from build123d import *

# Parameters (mm, degrees)
F0_W     = 181
F0_H     = 181
F0_W_2   = 20
F0_H_2   = 120
F1_DEPTH = 3


with BuildPart() as f1:
    # F0 (on Right) → F1 (new body)
    with BuildSketch(Plane.YZ):
        Rectangle(F0_W, F0_H)
        Polygon((8.017361, -22.155164), (10.511788, -22.155164), (11.657102, -24.445793), (13.264574, -44.539195), (13.264574, -24.155164), (19.664574, -24.155164), (19.664574, -27.155164), (24.664574, -27.155164), (24.664574, -72.955163), (3.864575, -72.955163), (3.864575, -27.155164), (8.864575, -27.155164), (8.864575, -24.955163), (6.617362, -24.955163), align=None, mode=Mode.SUBTRACT)
        Polygon((31.895746, -73.251659), (31.895746, -27.251661), (36.895746, -27.251661), (36.895746, -25.251659), (34.586729, -25.251659), (36.086728, -22.251661), (38.70476, -22.251661), (39.886403, -24.614947), (41.395744, -43.481709), (41.395744, -24.251661), (47.895743, -24.251661), (47.895743, -27.251661), (52.895743, -27.251661), (52.895743, -73.251659), align=None, mode=Mode.SUBTRACT)
        Polygon((73.728273, -23.606915), (73.728273, -26.606915), (78.728273, -26.606915), (78.728273, -72.806911), (57.528277, -72.806911), (57.528277, -26.606915), (62.528277, -26.606915), (62.528277, -24.806911), (60.157458, -24.806911), (61.757456, -21.606915), (64.499095, -21.606915), (65.717066, -24.042858), (67.128275, -41.682975), (67.128275, -23.606915), align=None, mode=Mode.SUBTRACT)
        with Locations((-69.899997, 23.899991)):
            Rectangle(F0_W_2, F0_H_2, mode=Mode.SUBTRACT)
        Polygon((-51.186814, -46.700009), (-51.186814, 83.899991), (-33.861232, 83.899991), (-33.861232, 73.899991), (-40.861232, 73.899991), (-40.861232, 63.999991), (-33.400224, 63.999991), (-33.400224, 53.799991), (-40.861232, 53.799991), (-40.861232, 44.099991), (-33.300224, 44.099991), (-33.300224, 33.699991), (-40.861232, 33.699991), (-40.861232, 24.199991), (-33.200224, 24.199991), (-33.200224, 13.599991), (-40.861232, 13.599991), (-40.861232, 4.299991), (-32.686683, 4.299991), (-32.686683, -6.500009), (-40.861232, -6.500009), (-40.861232, -15.600009), (-31.84899, -15.600009), (-31.84899, -26.600009), (-40.861232, -26.600009), (-40.861232, -35.500009), (-31.998828, -35.500009), (-31.998828, -46.700009), align=None, mode=Mode.SUBTRACT)
        Polygon((-7.774414, 73.899968), (-14.774414, 73.899968), (-14.774414, 63.799968), (-7.513406, 63.799968), (-7.513406, 53.999968), (-14.774414, 53.999968), (-14.774414, 43.699968), (-7.613406, 43.699968), (-7.613406, 34.099968), (-14.774414, 34.099968), (-14.774414, 23.599968), (-7.713406, 23.599968), (-7.713406, 14.199968), (-14.774414, 14.199968), (-14.774414, 3.499968), (-7.399865, 3.499968), (-7.399865, -5.700032), (-14.774414, -5.700032), (-14.774414, -16.600032), (-6.762172, -16.600032), (-6.762172, -25.600032), (-14.774414, -25.600032), (-14.774414, -36.700032), (-7.11201, -36.700032), (-7.11201, -45.500032), (-25.099996, -45.500032), (-25.099996, 83.899968), (-7.774414, 83.899968), align=None, mode=Mode.SUBTRACT)
        Polygon((19.364575, 31.999375), (19.364575, 28.999375), (24.364575, 28.999375), (24.364575, -16.200625), (4.164575, -16.200625), (4.164575, 28.999375), (9.164575, 28.999375), (9.164575, 31.799375), (7.102771, 31.799375), (8.202771, 33.999375), (10.326378, 33.999375), (11.362707, 31.926718), (13.164575, 9.403368), (13.164575, 31.999375), align=None, mode=Mode.SUBTRACT)
        Polygon((38.151176, 34.027429), (39.223833, 31.882114), (41.027569, 9.33542), (41.027569, 32.027429), (47.227569, 32.027429), (47.227569, 29.027429), (52.227569, 29.027429), (52.227569, -16.372571), (31.827568, -16.372571), (31.827568, 29.027429), (36.827568, 29.027429), (36.827568, 31.627429), (34.703961, 31.627429), (35.903962, 34.027429), align=None, mode=Mode.SUBTRACT)
        Polygon((73.428275, 32.017772), (73.428275, 29.017772), (78.428275, 29.017772), (78.428275, -16.582227), (57.828276, -16.582227), (57.828276, 29.017772), (62.828276, 29.017772), (62.828276, 31.417773), (60.642866, 31.417773), (61.942866, 34.017772), (64.313686, 34.017772), (65.422671, 31.799801), (67.128276, 10.479749), (67.128276, 32.017772), align=None, mode=Mode.SUBTRACT)
        Polygon((4.264574, 43.70002), (4.264574, 78.70002), (9.264574, 78.70002), (9.264574, 81.70002), (7.264574, 81.70002), (8.264574, 83.70002), (10.264574, 83.70002), (11.264574, 81.70002), (13.264574, 56.70002), (13.264574, 81.70002), (19.264574, 81.70002), (19.264574, 78.70002), (24.264574, 78.70002), (24.264574, 43.70002), align=None, mode=Mode.SUBTRACT)
        Polygon((32.027569, 42.248159), (32.027569, 78.70002), (37.027569, 78.70002), (37.027569, 81.70002), (35.027569, 81.70002), (36.027569, 83.70002), (38.027569, 83.70002), (39.027569, 81.70002), (41.027569, 56.70002), (41.027569, 81.70002), (47.027569, 81.70002), (47.027569, 78.70002), (52.027569, 78.70002), (52.027569, 42.248159), align=None, mode=Mode.SUBTRACT)
        Polygon((58.128275, 39.344446), (58.128275, 78.70002), (63.128275, 78.70002), (63.128275, 81.70002), (61.128275, 81.70002), (62.128275, 83.70002), (64.128275, 83.70002), (65.128275, 81.70002), (67.128275, 56.70002), (67.128275, 81.70002), (73.128275, 81.70002), (73.128275, 78.70002), (78.128275, 78.70002), (78.128275, 39.344446), align=None, mode=Mode.SUBTRACT)
    extrude(amount=F1_DEPTH)


solid = f1.part
The listing builds one solid part. Answer for the finished solid, in the listing's coordinates (mm). Coordinates: 2 decimals unless noted, no trailing zeros. Write each loop counter-clockwise with the first axis right and the second up, starting at its lowest first coordinate (ties: lowest second). Pieces come first, ordered by that corner, then holes. Notation, with made-up numbers: M -29.5,9.25 L -17.5,9.25 A16 ccw -17.5,17.25 Z; hole C 57.25,-36 d5. An arc over 180 degrees is marked long. Use one line per item in the form item = value.
Item 1: Find section C-C, the plane z = -67.5. Give the vertices of the cut face in (x, y).
Model answer:
outline = M 0,-90.5 L 3,-90.5 L 3,3.86 L 0,3.86 Z; M 0,24.66 L 3,24.66 L 3,31.9 L 0,31.9 Z; M 0,52.9 L 3,52.9 L 3,57.53 L 0,57.53 Z; M 0,78.73 L 3,78.73 L 3,90.5 L 0,90.5 Z
Item 2: Find section B-B, the plane z = 1. Give the vertices of the cut face in (x, y).
Model answer:
outline = M 0,-90.5 L 3,-90.5 L 3,-79.9 L 0,-79.9 Z; M 0,-59.9 L 3,-59.9 L 3,-51.19 L 0,-51.19 Z; M 0,-32.69 L 3,-32.69 L 3,-25.1 L 0,-25.1 Z; M 0,-7.4 L 3,-7.4 L 3,4.16 L 0,4.16 Z; M 0,24.36 L 3,24.36 L 3,31.83 L 0,31.83 Z; M 0,52.23 L 3,52.23 L 3,57.83 L 0,57.83 Z; M 0,78.43 L 3,78.43 L 3,90.5 L 0,90.5 Z
Item 3: Find the intervals of material crossed by probe 1 along Y at (x, z) = (1.95, -54); probe 2 along Z at (x, y) = (1.05, 58); probe 3 along Z at (x, y) = (1.75, 73), in increasing order.
Model answer:
probe_1 = -90.5 to 3.86, 24.66 to 31.9, 52.9 to 57.53, 78.73 to 90.5
probe_2 = -90.5 to -72.81, -26.61 to -16.58, 29.02 to 90.5
probe_3 = -90.5 to -72.81, -23.61 to -16.58, 32.02 to 39.34, 81.7 to 90.5
Item 4: Find section A-A, the plane y = -44.5. Give the vertices of the cut face in (x, z), plus the area to 3 significant figures.
Model answer:
outline = M 0,-90.5 L 3,-90.5 L 3,-46.7 L 0,-46.7 Z; M 0,83.9 L 3,83.9 L 3,90.5 L 0,90.5 Z
area = 151 mm2
Item 5: Find section D-D, the plane x = 1.7. Give the number of separate pieces and of enclosed holes in the cut face, plus the area to 3 significant figures.
Model answer:
separate_pieces = 1
enclosed_holes = 12
area = 18,500 mm2
